Read the model definition and answer for the solid it produces. Units are mm, in the model's axes. Coordinates: 2 decimals unless noted, no trailing zeros. Write each loop counter-clockwise with the first axis right and the second up, starting at its lowest first coordinate (ties: lowest second). Pieces come first, ordered by that corner, then holes.
(1) Given pin 1 (11 mm diameter, centred on x = 2.5, y = 27.5, fed in from +Z); pin 2 (1 mm diameter, centred on x = 0, z = 20, fed in from -Y); pin 3 (5 mm diameter, centred on x = 2.5, z = 122.25, fed in from +Y), each flat-ended and moving along its own axis, determine where each tip first touches the part or whether it passes through.
(2) The part is cut by section B-B, the plane x = -4. Determine the outline of the cut face in (y, z).
(3) The part is cut by section A-A, the plane y = -12.5. Determine the outline of the cut face in (x, z), and give its area (4 significant figures).
(4) The part is cut by section C-C, the plane z = 152.5. Determine the outline of the cut face in (x, y).
(5) The part is cut by section D-D, the plane y = 27. State how many separate pieces and enclosed holes the cut face has, and give its area (3 significant figures).
(6) Straight lines are drawn through the part: line 1 along Y through (x, z) = (7, 163); line 2 along Z through (x, y) = (-9.5, 31); line 3 along X through (y, z) = (27.5, -1.2). For each, find the intervals that lie inside material, in ascending order.
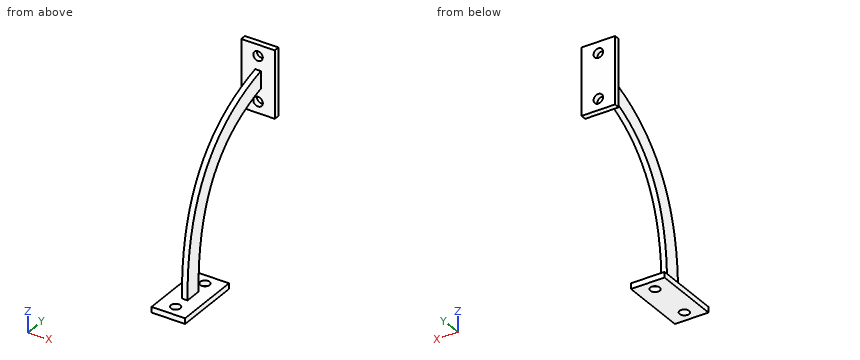
```python
from build123d import *

# Parameters (mm, degrees)
BOSS_EXTRUDE3_DEPTH = 5
SKETCH5_W           = 30
SKETCH5_H           = 60
SKETCH5_R           = 4.25
BOSS_EXTRUDE7_DEPTH = 5
SKETCH6_W           = 30
SKETCH6_H           = 60
SKETCH6_R           = 4.25
BOSS_EXTRUDE8_DEPTH = 5


# Read off the part's stored shape, not the designer's step: Boss-Extrude3
with BuildPart() as part:
    # Boss-Extrude3 outline → Boss-Extrude3 (new body)
    with BuildSketch(Plane(origin=(0, 0, 0), x_dir=(0, 0, -1), z_dir=(1, 0, 0))):
        with BuildLine():
            Line((-134.507952774, 100), (-150, 100))
            add(Edge.make_bspline(
                [(-150, 100), (-124.823277558, -2.14164181), (0, 0)],
                knots=[0, 0, 0, 1, 1, 1], degree=2))
            Line((0, 0), (0, 15))
            Line((0, 15), (-0.257322997, 14.997792667))
            add(Edge.make_bspline(
                [(-0.257322997, 14.997792667), (-22.513069097, 14.639377531), (-53.120235991, 19.679743273), (-74.17523554, 26.538598941), (-91.96421888, 36.076540514), (-106.790873123, 48.266354422), (-118.971580699, 63.298366178), (-130.328132656, 84.632434891), (-134.507952774, 100)],
                knots=[0, 0, 0, 0.1875, 0.3125, 0.4375, 0.5625, 0.6875, 0.8125, 0.98060163, 0.98060163, 0.98060163], degree=2))
        make_face()
    extrude(amount=BOSS_EXTRUDE3_DEPTH)

    # Sketch5 → Boss-Extrude7 (add)
    with BuildSketch(Plane(origin=(0, 100, 0), x_dir=(1, 0, 0), z_dir=(0, 1, 0))):
        with Locations((2.5, -142.253976387)):
            Rectangle(SKETCH5_W, SKETCH5_H)
        with Locations(Location((2.5, -162.253976387, 0), (0, 0, 270))):
            Circle(SKETCH5_R, mode=Mode.SUBTRACT)
        with Locations(Location((2.5, -122.253976387, 0), (0, 0, 90))):
            Circle(SKETCH5_R, mode=Mode.SUBTRACT)
    extrude(amount=BOSS_EXTRUDE7_DEPTH)

    # Sketch6 → Boss-Extrude8 (add)
    with BuildSketch(Plane(origin=(0, 0, 0), x_dir=(-1, 0, 0), z_dir=(0, 0, -1))):
        with Locations((-2.5, 7.5)):
            Rectangle(SKETCH6_W, SKETCH6_H)
        with Locations(Location((-2.5, 27.5, 0), (0, 0, 90))):
            Circle(SKETCH6_R, mode=Mode.SUBTRACT)
        with Locations(Location((-2.5, -12.5, 0), (0, 0, 90))):
            Circle(SKETCH6_R, mode=Mode.SUBTRACT)
    extrude(amount=BOSS_EXTRUDE8_DEPTH)


solid = part.part
```
Computed:
1. pin 1: stops at z = 111.73
1. pin 2: stops at y = 0.33
1. pin 3: stops at y = 74.19
2. outline: (-22.5, -5) - (37.5, -5) - (37.5, 0) - (-22.5, 0) - close; (100, 112.25) - (105, 112.25) - (105, 172.25) - (100, 172.25) - close
3. outline: (-12.5, -5) - (-1.75, -5) - (-1.75, 0) - (-12.5, 0) - close; (6.75, -5) - (17.5, -5) - (17.5, 0) - (6.75, 0) - close
3. area: 107.5 mm2
4. outline: (-12.5, 100) - (17.5, 100) - (17.5, 105) - (-12.5, 105) - close
5. separate pieces: 3
5. enclosed holes: 0
5. area: 259 mm2
6. line 1: y = 100 to 105
6. line 2: z = -5 to 0
6. line 3: x = -12.5 to -1.75, 6.75 to 17.5
